Autodesk Inventor part; units mm, degrees
ref_plane "YZ Plane" through (0, 0, 0) normal (1, 0, 0) x (0, 1, 0)
ref_plane "XZ Plane" through (0, 0, 0) normal (0, 1, 0) x (-1, 0, 0)
ref_plane "XY Plane" through (0, 0, 0) normal (0, 0, 1) x (1, 0, 0)
sketch "Sketch1" plane through (0, 0, 0) normal (1, 0, 0) x (0, 1, 0)
  line L0 (300, 0) -> (-300, 0)
  line L1 (-300, 0) -> (-300, -8.5)
  line L2 (-300, -8.5) -> (-163, -8.5)
  line L3 (300, -8.5) -> (300, 0)
  line L4 (185, -8.5) -> (185, -7.5)
  line L5 (185, -7.5) -> (184, -7.5)
  line L6 (184, -7.5) -> (184, -8.5)
  line L7 (-162, -7.5) -> (-163, -7.5)
  line L8 (-163, -7.5) -> (-163, -8.5)
  line L9 (-163, -8.5) -> (-162, -8.5) construction
  line L10 (-162, -8.5) -> (-162, -7.5)
  line L11 (220, -8.5) -> (300, -8.5) construction
  line L12 (300, -8.5) -> (220, -8.5) construction
  line L13 (220, -8.5) -> (220, -9.5)
  line L14 (220, -9.5) -> (300, -9.5)
  line L15 (300, -9.5) -> (300, -8.5)
  line L16 (184, -8.5) -> (185, -8.5) construction
  line L17 (185, -8.5) -> (220, -8.5)
  line L18 (-162, -8.5) -> (184, -8.5)
  line L19 (-163, -8.5) -> (-162, -8.5) construction
  point P0 (0, 0)
  point P1 (0, 0)
  point P2 (-163, -8.5)
  point P3 (-162, -8.5)
  dimension "d0" = 600
  dimension "d1" = 8.5
  dimension "d2" = 1
  dimension "d3" = 1
  dimension "d4" = 115
  dimension "d6" = 1
  dimension "d7" = 1
  dimension "d8" = 462
  dimension "d11" = 1
  dimension "d12" = 80
revolve "Revolution1" add sketch "Sketch1" angle 360 about axis through (0, 300, 0) along (0, -1, 0)
equation "\"d6\" = d2"
equation "\"d7\" = d3"
properties part number "Вал"
The listing builds one solid part. Answer for the finished solid, in the listing's coordinates (mm). A direction names the side the tool comes from. Round coordinates to 2 decimals unless told otherwise and drop trailing zeros. Loops run counter-clockwise (first coordinate to the right, second up) from the corner with the lowest first, then second, coordinate; pieces in that order, holes last. Notation, with made-up numbers: M 25.5,45.5 L 34.5,45.5 A18 ccw 34.5,58.5 Z; hole C -28.5,40 d3. An arc over 180 degrees is marked long. Return JSON: item names as keys, results as strings.
Q1. Find section B-B, the plane z = 0. Determine the outline of the cut face in (x, y).
Results list:
{"outline": "M -9.5,220 L -8.5,220 L -8.5,185 L -7.5,185 L -7.5,184 L -8.5,184 L -8.5,-162 L -7.5,-162 L -7.5,-163 L -8.5,-163 L -8.5,-300 L 8.5,-300 L 8.5,-163 L 7.5,-163 L 7.5,-162 L 8.5,-162 L 8.5,184 L 7.5,184 L 7.5,185 L 8.5,185 L 8.5,220 L 9.5,220 L 9.5,300 L -9.5,300 Z"}
Q2. Find section A-A, the plane x = 0. Determine the outline of the cut face in (y, z), plus the area to 3 significant figures.
Results list:
{"outline": "M -300,-8.5 L -163,-8.5 L -163,-7.5 L -162,-7.5 L -162,-8.5 L 184,-8.5 L 184,-7.5 L 185,-7.5 L 185,-8.5 L 220,-8.5 L 220,-9.5 L 300,-9.5 L 300,9.5 L 220,9.5 L 220,8.5 L 185,8.5 L 185,7.5 L 184,7.5 L 184,8.5 L -162,8.5 L -162,7.5 L -163,7.5 L -163,8.5 L -300,8.5 Z", "area": "10,400 mm2"}
Q3. Find the intervals of material crossed by line 1 along Y through (x, z) = (8.5, -2.75); line 2 along Z through (x, y) = (-1.25, -47.5); line 3 along X through (y, z) = (25, 4), in increasing order. Write a range as from..to.
Results list:
{"line 1": "y = 220..300", "line 2": "z = -8.41..8.41", "line 3": "x = -7.5..7.5"}
Q4. Each of these flat-tipped pins is pushed along its axis until it touches: pin 1 Ø1 at (x, y) = (5, -107.5) entering from -Z; pin 2 Ø4 at (x, y) = (-5, 215.5) entering from +Z; pin 3 Ø10 at (y, z) = (-196, 4) entering from +X. Where does it stop, or does it pass through?
Results list:
{"pin 1": "stops at z = -7.21", "pin 2": "stops at z = 7.95", "pin 3": "stops at x = 8.5"}
Q5. Find section D-D, the plane y = -41.5. Determine the outline of the cut face in (x, z).
Results list:
{"outline": "C 0,0 d17"}
Q6. Which of the six approach directions +Z, -Z, +X, -X, +Y, -Y give full straight-line access (tool end or side, diameter ignored) to faces 1 (the face through (-7.167, -230.541, -4.57)), 2 (the face through (-8, 184, 0)), 3 (the face through (0, -300, 0))?
Results list:
{"face 1": "-Y", "face 2": "none", "face 3": "+Z, -Z, +X, -X, -Y"}
Q7. Find section C-C, the plane y = 233. Determine the outline of the cut face in (x, z), plus the area to 3 significant figures.
Results list:
{"outline": "C 0,0 d19", "area": "284 mm2"}
